from build123d import *

# Parameters (mm, degrees)
SKETCH_1_W                 = 200
SKETCH_1_H                 = 73.5
EXTRUDE_1_DEPTH            = 3
SKETCH_2_R                 = 2.6
CUT_EXTRUDE_2_DEPTH        = 107.581248351
PATTERN_LINEAR_1_COUNT     = 5
PATTERN_LINEAR_1_PITCH     = 22
PATTERN_LINEAR_1_COL_COUNT = 5
PATTERN_LINEAR_1_COL_PITCH = 22
CUT_EXTRUDE_3_DEPTH        = 107.581248351
CUT_EXTRUDE_3_DEPTH_BACK   = 107.581248351
SKETCH_3_W                 = 3
SKETCH_3_H                 = 73.5
CUT_EXTRUDE_4_DEPTH        = 104.771684481
CUT_EXTRUDE_4_DEPTH_BACK   = 104.771684481


with BuildPart() as part:
    # 草图1 → 凸台-拉伸1 (new body)
    with BuildSketch(Plane.XY):
        Rectangle(SKETCH_1_W, SKETCH_1_H)
    extrude(amount=EXTRUDE_1_DEPTH)

    # 草图2 → 切除-拉伸2 (cut, symmetric)
    with BuildSketch(Plane.XY.offset(3)):
        with Locations((0, 26.75)):
            Circle(SKETCH_2_R)
    cut_extrude_2 = extrude(amount=CUT_EXTRUDE_2_DEPTH, both=True, mode=Mode.SUBTRACT)

    # 阵列(线性)1: 切除-拉伸2 ×5
    with Locations(*[(i * PATTERN_LINEAR_1_PITCH, 0, 0) for i in range(1, PATTERN_LINEAR_1_COUNT)]):
        add(cut_extrude_2, mode=Mode.SUBTRACT)

    # 阵列(线性)1 col: 切除-拉伸2 ×5
    with Locations(*[(-i * PATTERN_LINEAR_1_COL_PITCH, 0, 0) for i in range(1, PATTERN_LINEAR_1_COL_COUNT)]):
        add(cut_extrude_2, mode=Mode.SUBTRACT)

    # 草图3 → 切除-拉伸3 (cut, two sides: drawn at the far end of the back side and taken through both)
    with BuildSketch(Plane.XY.offset(3).offset(-CUT_EXTRUDE_3_DEPTH_BACK)):
        with Locations((-98.5, 0)):
            Rectangle(SKETCH_3_W, SKETCH_3_H)
        with Locations((98.5, 0)):
            Rectangle(SKETCH_3_W, SKETCH_3_H)
    extrude(amount=CUT_EXTRUDE_3_DEPTH + CUT_EXTRUDE_3_DEPTH_BACK, mode=Mode.SUBTRACT)

    # 草图4 → 切除-拉伸4 (cut, two sides: drawn at the far end of the back side and taken through both)
    with BuildSketch(Plane.XY.offset(3).offset(-CUT_EXTRUDE_4_DEPTH_BACK)):
        with BuildLine():
            Line((63.303207355, -36.75), (97, -36.75))
            Line((97, -36.75), (97, 36.75))
            add(Edge.make_bspline(
                [(63.303207355, -36.75), (92.189094157, -6.525878678), (97, 36.75)],
                knots=[0, 0, 0, 1, 1, 1], degree=2))
        make_face()
    extrude(amount=CUT_EXTRUDE_4_DEPTH + CUT_EXTRUDE_4_DEPTH_BACK, mode=Mode.SUBTRACT)


solid = part.part
Could you check a few things on this model? Use its own coordinates, in mm. Coordinates: 2 decimals unless noted, no trailing zeros. Order: outer loops, then holes, each group sorted by start corner. A loop starts at its lowest first (then second) coordinate and runs counter-clockwise, first axis right, second up. Notation, with made-up numbers: (-30, -7) - (16, -7) arc R14 cw to (16, 3) - close; hole circle Ø6 at (-39.75, -16.75). An arc over 180 degrees is marked (long way). Answer in a Markdown table with one row per item. Add a question column.
(1) Will these pins go through, and if not, where does the flat tip stop? pin 1 (3 mm diameter, centred on x = 0, y = 26.75, fed in from -Z); pin 2 (6 mm diameter, centred on x = 44, y = 26.75, fed in from +Z).
(2) If we section it at A-A, the plane x = -88: Please give me the cut outline in (y, z).
(3) I need wall thicknesses on L1, parallel to Y at x = -66, z = 1.95; L2, parallel to Y at x = 88, z = 0.85; L3, parallel to X at y = 8.5, z = 1.55. Which ranges of each line are inside material? Lowest first, please.
(4) If we mould it in two halves opening along Y, with no side actions, what happens to faces 1 (the face through (-1, 1, 3)), 2 (the face through (63.403, 26.864, 1.521))? For each: released by +Y, released by -Y, zero draft, split by the parting line, or undercut.
(5) If we section it at B-B, the plane z = 1.2: State how many separate pieces and enclosed holes the cut face has, then the cut area to 3 significant figures.
Results are:
| question | item | result |
|---|---|---|
| 1 | pin 1 | passes through |
| 1 | pin 2 | stops at z = 3 |
| 2 | outline | (-36.75, 0) - (24.15, 0) - (24.15, 3) - (-36.75, 3) - close; (29.35, 0) - (36.75, 0) - (36.75, 3) - (29.35, 3) - close |
| 3 | L1 | y = -36.75 to 24.15, 29.35 to 36.75 |
| 3 | L2 | y = 0.94 to 24.15, 29.35 to 36.75 |
| 3 | L3 | x = -97 to 90.83 |
| 4 | face 1 | zero draft |
| 4 | face 2 | undercut |
| 5 | separate pieces | 1 |
| 5 | enclosed holes | 9 |
| 5 | area | 13,200 mm2 |
